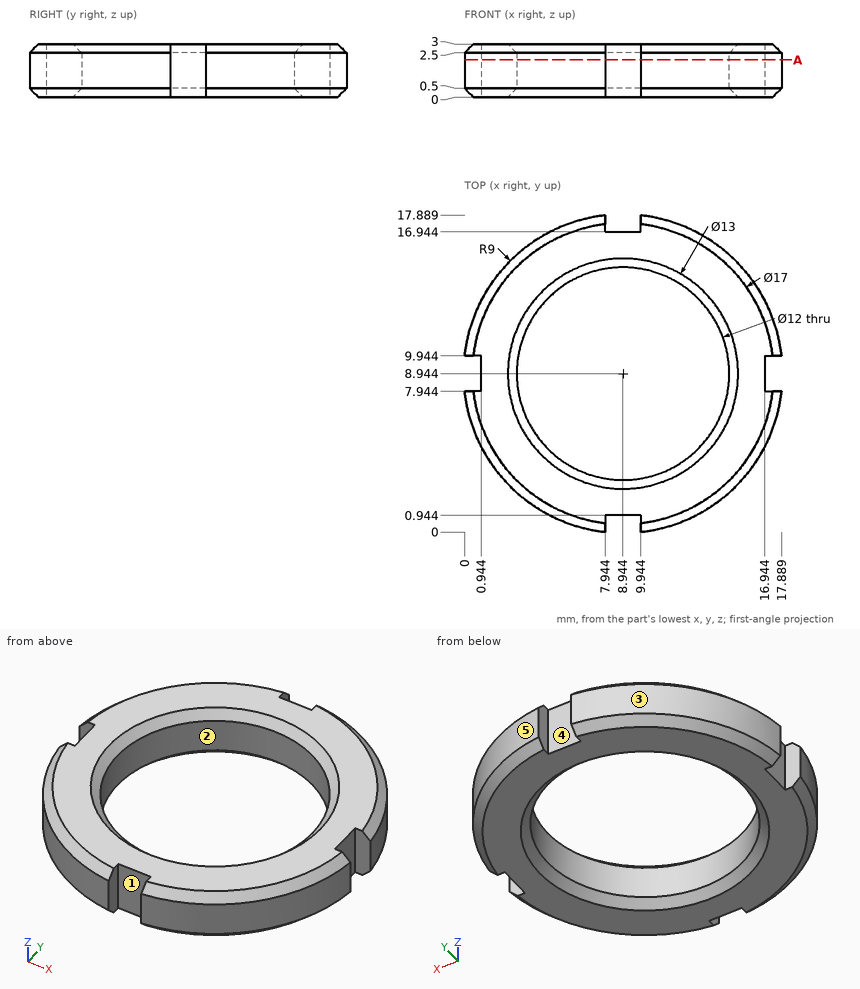
Check sheet for the drawn part. Datum: minimum x, y, z corner. Units: mm. A direction names the side the tool comes from. Round coordinates to 2 decimals unless told otherwise and drop trailing zeros. Order: outer loops, then holes, each group sorted by start corner. A loop starts at its lowest first (then second) coordinate and runs counter-clockwise, first axis right, second up. Notation, with made-up numbers: (34, 18.5) -> (71, 18.5) arc R8 cw to (71, 29.5) -> close; hole circle Ø4 at (-15, 0.5). An arc over 180 degrees is marked (long way). Put each result on its own line as item: value. Start each with the question number.
(1) Section check A-A (z = 2.1). Enter the section's corners in (x, y) (1 decimal).
(2) Depth check by flat-ended pin: pin 1 Ø1.6 at (x, z) = (8.5, 1) entering from -Y; pin 2 Ø1 at (y, z) = (0.5, 2) entering from -X (1 decimal); pin 3 Ø1 at (y, z) = (0.5, 1) entering from +X (1 decimal); pin 4 Ø1.5 at (x, z) = (15.5, 0.5) entering from +Y. Enter the tip coordinate at first touch or a pass-through.
(3) Material ranges on line 1 along Y through (x, z) = (9.5, 2.35) (1 decimal); line 2 along Y through (x, z) = (8.75, 1.7) (1 decimal); line 3 along X through (y, z) = (17.25, 1.55) (1 decimal), recorded low to high.
(4) Tool access check on the marked faces 4 and 5. Record the directions out of +Z, -Z, +X, -X, +Y, -Y that give a thin tool (end or side, any length) a straight path to the whole face; none if there is none.
(5) Draft check along Y on the marked faces 1, 2 and 3. Enter one of: +Y half, -Y half, draft (parallel to the pull), parting line (faces both ways), or undercut.
Completed:
1. outline: (0, 7.9) arc R9 ccw to (7.9, 0) -> (7.9, 0.9) -> (9.9, 0.9) -> (9.9, 0) arc R9 ccw to (17.9, 7.9) -> (16.9, 7.9) -> (16.9, 9.9) -> (17.9, 9.9) arc R9 ccw to (9.9, 17.9) -> (9.9, 16.9) -> (7.9, 16.9) -> (7.9, 17.9) arc R9 ccw to (0, 9.9) -> (0.9, 9.9) -> (0.9, 7.9) -> close; hole circle Ø12 at (8.9, 8.9)
2. pin 1: stops at y = 0
2. pin 2: stops at x = 4.7
2. pin 3: stops at x = 13.2
2. pin 4: stops at y = 15.82
3. line 1: y = 0.9 to 3, 14.9 to 16.9
3. line 2: y = 0.9 to 2.9, 14.9 to 16.9
3. line 3: x = 5.5 to 7.9, 9.9 to 12.4
4. face 4: +Z, -Z, +Y
4. face 5: +Z, -Z, +X, +Y
5. face 1: -Y half
5. face 2: undercut
5. face 3: +Y half
